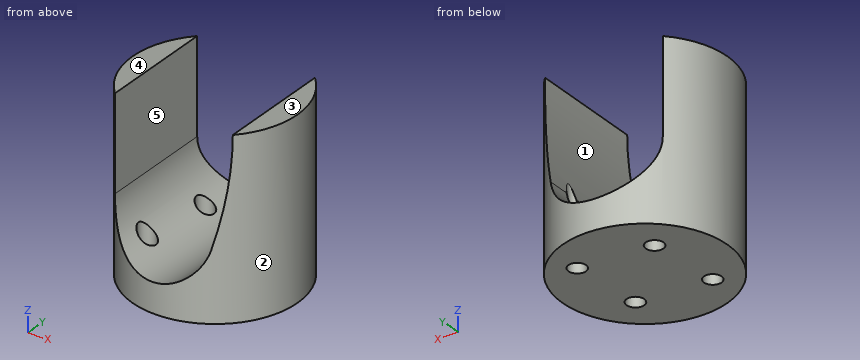
```python
from build123d import *

# Parameters (mm, degrees)
F0_R          = 14
F0_R_2        = 1.5
F1_DEPTH      = 30
F3_DEPTH      = 25
F3_DEPTH_BACK = 25


with BuildPart() as f1:
    # F0 (on Top) → F1 (new body)
    with BuildSketch(Plane.XY):
        Circle(F0_R)
        with Locations((-6.7175144213, -6.7175144213)):
            Circle(F0_R_2, mode=Mode.SUBTRACT)
        with Locations((5.6568542495, -5.6568542495)):
            Circle(F0_R_2, mode=Mode.SUBTRACT)
        with Locations((-5.6568542495, 5.6568542495)):
            Circle(F0_R_2, mode=Mode.SUBTRACT)
        with Locations((6.7175144213, 6.7175144213)):
            Circle(F0_R_2, mode=Mode.SUBTRACT)
    extrude(amount=F1_DEPTH)

    # F2 (on Front) → F3 (cut, two sides)
    with BuildSketch(Plane.XZ) as f3_sk:
        with BuildLine():
            Line((10, 30), (-10, 30))
            Line((-10, 30), (-10, 13.9895361748))
            ThreePointArc((-10, 13.9895361748), (-2.136238911, 5.0707699432), (7.6971068467, 11.7557112868))
            ThreePointArc((7.6971068467, 11.7557112868), (9.4220015712, 20.8054719055), (10, 30))
        make_face()
    extrude(amount=-F3_DEPTH, mode=Mode.SUBTRACT)
    extrude(f3_sk.sketch, amount=F3_DEPTH_BACK, mode=Mode.SUBTRACT)


solid = f1.part
```
Part model, mm, in its own coordinate system. Face numbers are marked on the shaded views. A direction names the side the tool comes from. Round coordinates to 2 decimals unless told otherwise and drop trailing zeros. Loops run counter-clockwise (first coordinate to the right, second up) from the corner with the lowest first, then second, coordinate; pieces in that order, holes last.
1. Flat gauge pins, fed straight in: pin 1 (12 mm diameter, centred on y = -10, z = 8, fed in from -X); pin 2 (1.5 mm diameter, centred on x = 0.5, y = 5.5, fed in from +Z); pin 3 (4 mm diameter, centred on y = -9, z = 22.5, fed in from +X). Where does each tip first touch, or does it go through?
Solutions:
pin 1: stops at x = -13.42
pin 2: stops at z = 5.29
pin 3: stops at x = 12.12
2. Slice it at C-C (x = 1). Give the cut face in (y, z).
Solutions:
outline: (-13.96, 0) - (13.96, 0) - (13.96, 5.23) - (-13.96, 5.23) - close
3. 3-axis set-ups, long thin cutter, end or side, ignore diameter. For the marked faces 4 and 5: which of +Z, -Z, +X, -X, +Y, -Y reach the whole face in a straight line?
Solutions:
face 4: +Z, +X, -X, +Y, -Y
face 5: +Z, +Y, -Y
4. Slice it at A-A (y = 0). Give the cut face in (x, z).
Solutions:
outline: (-14, 0) - (14, 0) - (14, 30) - (10, 30) arc R73.42 cw to (7.7, 11.76) arc R8.99 cw to (-10, 13.99) - (-10, 30) - (-14, 30) - close
5. Slice it at D-D (y = -8.75). Give the cut face in (x, z), and give its area (3 significant figures).
Solutions:
outline: (-10.93, 0) - (10.93, 0) - (10.93, 30) - (10, 30) arc R73.42 cw to (7.7, 11.76) arc R8.99 cw to (-10, 13.99) - (-10, 30) - (-10.93, 30) - close
area: 218 mm2
6. Two-plate mould, pull along X, no slides. Class the marked faces 1, 2 and 3: pulls with the +X half, pulls with the -X half, needs draft (parallel to the pull), parting line crosses it, or undercut.
Solutions:
face 1: undercut
face 2: parting line crosses it
face 3: needs draft
7. Drill centre lines: line 1 along X through (y, z) = (-2.75, 15.5); line 2 along X through (y, z) = (3.75, 14); line 3 along Z through (x, y) = (3.5, 0.5). Where is each one in solid material? Low to high.
Solutions:
line 1: x = -13.73 to -10, 8.55 to 13.73
line 2: x = -13.49 to -10, 8.24 to 13.49
line 3: z = 0 to 6.21
8. Slice it at B-B (x = -6). Give the cut face in (y, z), and give its area (3 significant figures).
Solutions:
outline: (-12.65, 0) - (-8.03, 0) - (-8.03, 6.51) - (-12.65, 6.51) - close; (-5.4, 0) - (4.2, 0) - (4.2, 6.51) - (-5.4, 6.51) - close; (7.12, 0) - (12.65, 0) - (12.65, 6.51) - (7.12, 6.51) - close
area: 129 mm2
